Part print with two shaded views. Sizes in mm from the minimum x, y, z corner. A direction names the side the tool comes from. Round coordinates to 2 decimals unless told otherwise and drop trailing zeros. Write each loop counter-clockwise with the first axis right and the second up, starting at its lowest first coordinate (ties: lowest second). Pieces come first, ordered by that corner, then holes.
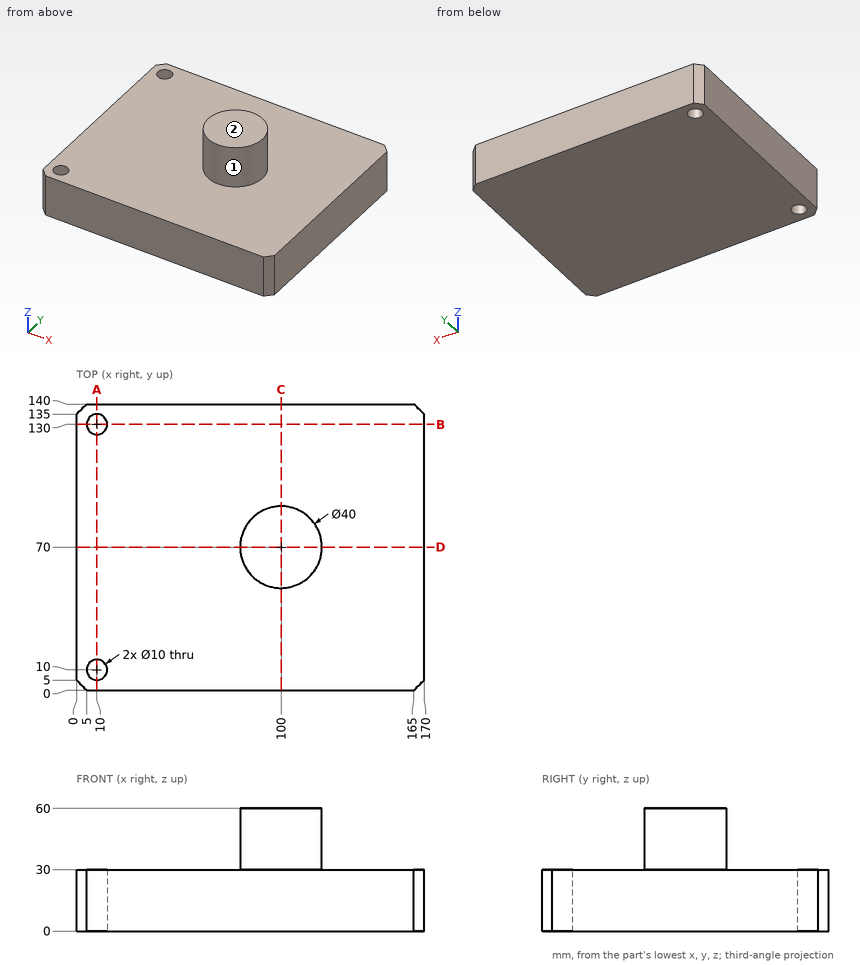
Q1. Drop flat-ended pins along their axis: pin 1 (11.5 mm diameter, centred on x = 10, y = 130, fed in from +Z); pin 2 (1.5 mm diameter, centred on x = 53.5, y = 109, fed in from -Z); pin 3 (9 mm diameter, centred on x = 10, y = 10, fed in from +Z); pin 4 (12 mm diameter, centred on x = 84, z = 40.5, fed in from -Y). Give the stop position or say it passes through.
Values follow:
pin 1: stops at z = 30
pin 2: stops at z = 0
pin 3: passes through
pin 4: stops at y = 52.68
Q2. Cut at D-D on y = 70. Write the cut outline in (x, z).
Values follow:
outline: (0, 0) - (170, 0) - (170, 30) - (120, 30) - (120, 60) - (80, 60) - (80, 30) - (0, 30) - close
Q3. Cut at A-A on x = 10. Write the cut outline in (y, z).
Values follow:
outline: (0, 0) - (5, 0) - (5, 30) - (0, 30) - close; (15, 0) - (125, 0) - (125, 30) - (15, 30) - close; (135, 0) - (140, 0) - (140, 30) - (135, 30) - close
Q4. Which spindle directions (+Z, -Z, +X, -X, +Y, -Y) get a long thin tool onto all of the face, cutting with end or side? Do the marked faces 1 and 2. Say none if no direction does.
Values follow:
face 1: +Z
face 2: +Z, +X, -X, +Y, -Y
Q5. Cut at B-B on y = 130. Write the cut outline in (x, z), plus the area to 3 significant figures.
Values follow:
outline: (0, 0) - (5, 0) - (5, 30) - (0, 30) - close; (15, 0) - (170, 0) - (170, 30) - (15, 30) - close
area: 4,800 mm2
Q6. Cut at C-C on x = 100. Write the cut outline in (y, z), plus the area to 3 significant figures.
Values follow:
outline: (0, 0) - (140, 0) - (140, 30) - (90, 30) - (90, 60) - (50, 60) - (50, 30) - (0, 30) - close
area: 5,400 mm2
Q7. Wall check: L1, parallel to Y at x = 10, z = 11; L2, parallel to X at y = 130, z = 16; L3, parallel to Z at x = 78.5, y = 82. Give the ranges that are in metal, low to high.
Values follow:
L1: y = 0 to 5, 15 to 125, 135 to 140
L2: x = 0 to 5, 15 to 170
L3: z = 0 to 30
